Geometry check sheet. Reference: the model listing, model coordinates, mm. Face numbers are marked on the shaded views. A direction names the side the tool comes from. Round coordinates to 2 decimals unless told otherwise and drop trailing zeros. Loops run counter-clockwise (first coordinate to the right, second up) from the corner with the lowest first, then second, coordinate; pieces in that order, holes last. Notation, with made-up numbers: (21, 70.5) - (60, 70.5) arc R27 ccw to (60, 100.5) - close; hole circle Ø10 at (89.5, -6.5). An arc over 180 degrees is marked (long way). Answer as CSV lines item,"result". Start each with the question number.
1) Cross-section at A-A on x = 0. Record the boundary of the cut face in (y, z), and give its area (3 significant figures).
2) Cross-section at B-B on y = 0. Record the boundary of the cut face in (x, z).
3) Cross-section at D-D on z = -9.5. Record the boundary of the cut face in (x, y), and give its area (3 significant figures).
4) Access from +Z, -Z, +X, -X, +Y, -Y to the whole of each face (thin tool, end or side, straight path). Record for the marked faces 5 and 6.
5) Cross-section at C-C on z = -16. Record the boundary of the cut face in (x, y).
6) Draft check along Y on the marked faces 1, 2, 3 and 4. Enter one of: released by +Y, released by -Y, zero draft, split by the parting line, or undercut.
7) Depth check by flat-ended pin: P1, Ø1.9, axis at x = 25.58, y = 9.32, coming from the -Z side; P2, Ø6.5, axis at y = 3.5, z = -3.5, coming from the -X side; P3, Ø2, axis at y = 22, z = 3.5, coming from the -X side. Enter the tip coordinate at first touch or a pass-through.
8) Thickness scan on line 1 along Y through (x, z) = (0, -9); line 2 along Z through (x, y) = (18, -29.5); line 3 along X through (y, z) = (0, -17). Record the ranges inside material, lowest first.
from build123d import *

# Parameters (mm, degrees)
F0_R      = 39.37
F1_DEPTH  = 12.7
F2_T      = -2.54
F3_R      = 5.08
F4_R      = 2.54
F5_R      = 19.05
F6_DEPTH  = 25.4
F7_R      = 39.37
F7_R_2    = 1.0414
F7_R_3    = 1.016
F8_DEPTH  = 12.7
F9_R      = 39.37
F9_R_2    = 38.1
F10_DEPTH = 6.35


with BuildPart() as f1:
    # F0 (on Top) → F1 (new body)
    with BuildSketch(Plane.XY):
        Circle(F0_R)
    extrude(amount=F1_DEPTH)

    # F2
    f2_openings = [f1.faces().sort_by_distance(p)[0] for p in [
        (0, 0, 0),
    ]]
    offset(amount=F2_T, openings=f2_openings)

    # F3
    f3_edges = [f1.edges().sort_by_distance(p)[0] for p in [
        (-39.37, 0, 12.7),
    ]]
    fillet(f3_edges, radius=F3_R)

    # F4
    f4_edges = [f1.edges().sort_by_distance(p)[0] for p in [
        (-36.83, 0, 10.16),
    ]]
    fillet(f4_edges, radius=F4_R)

    # F5 (on face) → F6 (cut)
    with BuildSketch(Plane(origin=(0, 0, 10.16), x_dir=(1, 0, 0), z_dir=(0, 0, -1))):
        Circle(F5_R)
    extrude(amount=-F6_DEPTH, mode=Mode.SUBTRACT)

    # F7 (on face) → F8 (join)
    with BuildSketch(Plane(origin=(0, 0, 0), x_dir=(1, 0, 0), z_dir=(0, 0, -1))):
        Circle(F7_R)
        with BuildLine():
            ThreePointArc((18.923, -31.5969772447), (-29.1572661412, -22.5011717733), (-25.7682217594, 26.3144))
            Line((-25.7682217594, 26.3144), (18.923, 26.3144))
            Line((18.923, 26.3144), (18.923, -31.5969772447))
        make_face(mode=Mode.SUBTRACT)
        with Locations((25.5778, -9.3218)):
            Circle(F7_R_2, mode=Mode.SUBTRACT)
        with Locations((0, 28.3972)):
            Circle(F7_R_3, mode=Mode.SUBTRACT)
    extrude(amount=F8_DEPTH)

    # F9 (on face) → F10 (join)
    with BuildSketch(Plane(origin=(0, 0, -12.7), x_dir=(1, 0, 0), z_dir=(0, 0, -1))):
        Circle(F9_R)
        Circle(F9_R_2, mode=Mode.SUBTRACT)
    extrude(amount=F10_DEPTH)


solid = f1.part
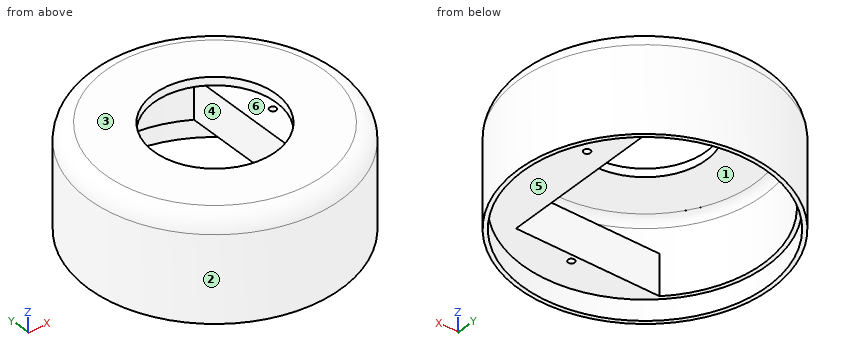
Answer block:
1,outline,"(-39.37, -19.05) - (-38.1, -19.05) - (-38.1, -12.7) - (-29.41, -12.7) - (-29.41, 0) - (-36.83, 0) - (-36.83, 7.62) arc R2.54 cw to (-34.29, 10.16) - (-19.05, 10.16) - (-19.05, 12.7) - (-34.29, 12.7) arc R5.08 ccw to (-39.37, 7.62) - close; (-27.38, -12.7) - (-26.31, -12.7) - (-26.31, 0) - (-27.38, 0) - close; (19.05, 10.16) - (34.29, 10.16) arc R2.54 cw to (36.83, 7.62) - (36.83, -12.7) - (38.1, -12.7) - (38.1, -19.05) - (39.37, -19.05) - (39.37, 7.62) arc R5.08 ccw to (34.29, 12.7) - (19.05, 12.7) - close"
1,area,"335 mm^2"
2,outline,"(-39.37, -19.05) - (-38.1, -19.05) - (-38.1, -12.7) - (-36.83, -12.7) - (-36.83, 7.62) arc R2.54 cw to (-34.29, 10.16) - (-19.05, 10.16) - (-19.05, 12.7) - (-34.29, 12.7) arc R5.08 ccw to (-39.37, 7.62) - close; (18.92, -12.7) - (38.1, -12.7) - (38.1, -19.05) - (39.37, -19.05) - (39.37, 7.62) arc R5.08 ccw to (34.29, 12.7) - (19.05, 12.7) - (19.05, 10.16) - (34.29, 10.16) arc R2.54 cw to (36.83, 7.62) - (36.83, 0) - (18.92, 0) - close"
3,outline,"circle Ø78.74 at (0, 0); hole (-25.77, -26.31) - (18.92, -26.31) - (18.92, 31.6) arc R36.83 ccw to start; hole circle Ø2.03 at (0, -28.4); hole circle Ø2.08 at (25.58, 9.32)"
3,area,"1,760 mm^2"
4,face 5,"-Z"
4,face 6,"none"
5,outline,"circle Ø78.74 at (0, 0); hole circle Ø76.2 at (0, 0)"
6,face 1,"undercut"
6,face 2,"split by the parting line"
6,face 3,"zero draft"
6,face 4,"undercut"
7,P1,"stops at z = 10.16"
7,P2,"stops at x = -39.37"
7,P3,"stops at x = -33.3"
8,line 1,"y = -39.37 to -29.41, -27.38 to -26.31, 36.83 to 39.37"
8,line 2,"z = -12.7 to 0, 10.15 to 12.69"
8,line 3,"x = -39.37 to -38.1, 38.1 to 39.37"
